Work out the finished part from the listing and answer in its coordinate system (mm). Face numbers are marked on the shaded views. A direction names the side the tool comes from. Give positions to 0.01 mm unless a question says otherwise; leave off trailing zeros. Loops run counter-clockwise (first coordinate to the right, second up) from the corner with the lowest first, then second, coordinate; pieces in that order, holes last. Notation, with made-up numbers: (2, 59.25) - (60, 59.25) arc R15 ccw to (60, 84.25) - close; hole circle Ø7 at (47, 59.5). An arc over 180 degrees is marked (long way). Use CSV: the item, a comma, the result in double quotes.
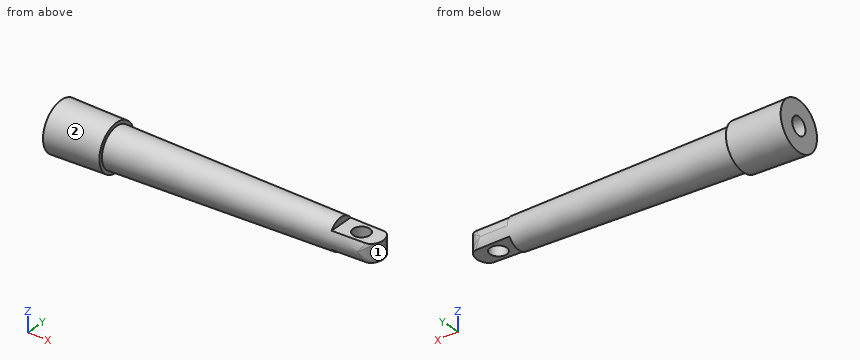
from build123d import *
from build123d.topology import SkipClean

# Parameters (mm, degrees)
BOSS_EXTRUDE1_DEPTH     = 1
CUT_EXTRUDE1_DEPTH      = 37.54772833504248
CUT_EXTRUDE1_DEPTH_BACK = 37.54772833504248
SKETCH4_R               = 0.9500000000000008
FILLET1_R               = 0.5
SKETCH5_R               = 1
CUT_EXTRUDE2_DEPTH      = 26.5


with BuildPart() as part:
    # Sketch1 → Revolve1 (revolve)
    with BuildSketch(Plane.XY, mode=Mode.PRIVATE) as revolve1_sk:
        Polygon((0, 0), (31.5, 0), (31.5, 1.7500000000000002), (6.25, 2.25), (6.25, 2.63), (-8.6e-16, 2.753762376237624), align=None)
    revolve(revolve1_sk.sketch.rotate(Axis((0, 0, 0), (1, 0, 0)), 90), axis=Axis((0, 0, 0), (1, 0, 0)))

    # Sketch2 → Boss-Extrude1 (add, symmetric)
    with BuildSketch(Plane.XY):
        with BuildLine():
            Line((31.5, 1.7500000000000002), (34.59438397289708, 1.6887250698436231))
            ThreePointArc((34.59438397289708, 1.6887250698436231), (36.250000000000384, 0), (34.59438397289708, -1.6887250698436231))
            Line((34.59438397289708, -1.6887250698436231), (31.5, -1.7500000000000002))
            Line((31.5, -1.7500000000000002), (31.5, 1.7500000000000002))
        make_face()
    extrude(amount=BOSS_EXTRUDE1_DEPTH, both=True)

    # Sketch3 → Cut-Revolve1 (revolve, cut)
    with SkipClean():  # the faces are left unmerged after this step: merging them gives an invalid solid
        with BuildSketch(Plane.XY):
            Polygon((31.5, 1.7500000000000002), (31.5, 3.02899348193033), (37.16046821617775, 3.02899348193033), (37.16046821617775, 1.6379115204717292), align=None)
        revolve(axis=Axis((31.5, 0, 0), (1, 0, 0)), mode=Mode.SUBTRACT)

    # Sketch4 → Cut-Extrude1 (cut, two sides: drawn at the far end of the back side and taken through both)
    with SkipClean():  # the faces are left unmerged after this step: merging them gives an invalid solid
        with BuildSketch(Plane.XY.offset(1).offset(-CUT_EXTRUDE1_DEPTH_BACK)):
            with Locations((33.800000000000416, 0)):
                Circle(SKETCH4_R)
        extrude(amount=CUT_EXTRUDE1_DEPTH + CUT_EXTRUDE1_DEPTH_BACK, mode=Mode.SUBTRACT)

    # Fillet1
    fillet1_edges = [part.edges().sort_by_distance(p)[0] for p in [
        (35.10948652987232, 1.5975016585971056, -0.5152035376774515),
        (35.109486521686094, -1.5975016606575614, -0.5152035294896175),
        (35.109486530948786, 1.5975016579572403, 0.5152035387541277),
        (35.10948652164611, -1.5975016610354238, 0.5152035294496282),
    ]]
    fillet(fillet1_edges, radius=FILLET1_R)

    # Sketch5 → Cut-Extrude2 (cut)
    with SkipClean():  # the faces are left unmerged after this step: merging them gives an invalid solid
        with BuildSketch(Plane.ZY):
            Circle(SKETCH5_R)
        extrude(amount=-CUT_EXTRUDE2_DEPTH, mode=Mode.SUBTRACT)


solid = part.part
Item 1: A cutting plane is placed at C-C on x = 13. Determine the outline of the cut face in (y, z).
Determined:
outline,"circle Ø4.23 at (0, 0); hole circle Ø2 at (0, 0)"
Item 2: A cutting plane is placed at A-A on x = 33.8. Determine the outline of the cut face in (y, z), and give its area (3 significant figures).
Determined:
outline,"(-1.38, -1) - (-0.95, -1) - (-0.95, 1) - (-1.38, 1) arc R1.7 ccw to start; (0.95, -1) - (1.38, -1) arc R1.7 ccw to (1.38, 1) - (0.95, 1) - close"
area,"2.60 mm²"
Item 3: For the marked faces 1 and 2, determine the directions among +Z, -Z, +X, -X, +Y, -Y from which every point of the face is accessible in a straight line to the end or side of a thin tool.
Determined:
face 1,"+Z, -Z, +X"
face 2,"+X"
Item 4: Find the intervals of material crossed by line 1 (Y direction, x = 33.8, z = 0.2); line 2 (X direction, y = 0, z = -0.2); line 3 (X direction, y = -2.1, z = -1), in increasing order.
Determined:
line 1,"y = -1.69 to -0.95, 0.95 to 1.69"
line 2,"x = 26.5 to 32.85, 34.75 to 36.25"
line 3,"x = 0 to 6.25"
Item 5: Given P1, Ø1, axis at x = 20, y = 1, coming from the -Z side; P2, Ø3, axis at x = 27.5, y = 1.5, coming from the +Z side; P3, Ø2.5, axis at y = 1, z = -1, coming from the +X side; P4, Ø2.5, axis at x = 33.8, y = 0, coming from the +Z side, each flat-ended and moving along its own axis, determine where each tip first touches the part or whether it passes through.
Determined:
P1,"stops at z = -1.91"
P2,"stops at z = 1.84"
P3,"stops at x = 36.25"
P4,"stops at z = 1"
Item 6: A cutting plane is placed at B-B on x = 3.5. Determine the outline of the cut face in (y, z), and give its area (3 significant figures).
Determined:
outline,"circle Ø5.37 at (0, 0); hole circle Ø2 at (0, 0)"
area,"19.5 mm²"
